```python
from build123d import *

# Parameters (mm, degrees)
BOSS_EXTRUDE1_DEPTH      = 85
BOSS_EXTRUDE1_DEPTH_BACK = 30
CUT_EXTRUDE1_DEPTH       = 134.120246394
CUT_EXTRUDE1_DEPTH_BACK  = 134.120246394
SKETCH3_R                = 20
CHAMFER1_SIZE            = 10
CHAMFER2_SIZE            = 60


with BuildPart() as part:
    # Sketch2 → Boss-Extrude1 (new, two sides: drawn at the far end of the back side and taken through both)
    with BuildSketch(Plane.XY.offset(-BOSS_EXTRUDE1_DEPTH_BACK)):
        Polygon((0, 0), (-50, 0), (-50, 80), (-64, 80), (-64, -8), (14, -8), (14, 80), (0, 80), align=None)
    extrude(amount=BOSS_EXTRUDE1_DEPTH + BOSS_EXTRUDE1_DEPTH_BACK)

    # Sketch3 → Cut-Extrude1 (cut, two sides: drawn at the far end of the back side and taken through both)
    with BuildSketch(Plane(origin=(0, 0, 0), x_dir=(0, 0, -1), z_dir=(1, 0, 0)).offset(-CUT_EXTRUDE1_DEPTH_BACK)):
        with Locations(Location((0, 50, 0), (0, 0, 90))):
            Circle(SKETCH3_R)
    extrude(amount=CUT_EXTRUDE1_DEPTH + CUT_EXTRUDE1_DEPTH_BACK, mode=Mode.SUBTRACT)

    # Chamfer1
    chamfer1_edges = [part.edges().sort_by_distance(p)[0] for p in [
        (-50, 0, 27.5),
        (0, 0, 27.5),
    ]]
    chamfer(chamfer1_edges, length=CHAMFER1_SIZE)

    # Chamfer2
    chamfer2_edges = [part.edges().sort_by_distance(p)[0] for p in [
        (-57, 80, 85),
        (7, 80, 85),
    ]]
    chamfer(chamfer2_edges, length=CHAMFER2_SIZE)


solid = part.part
```
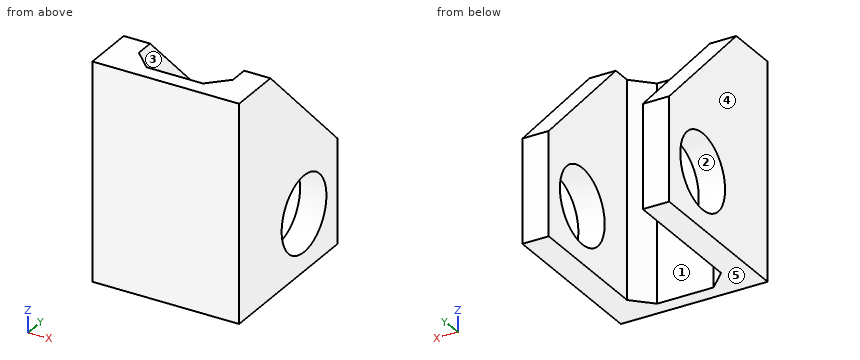
Design review of the part built by this model. Coordinates are the model's own, in mm. Face numbers are marked on the shaded views. A direction names the side the tool comes from. Give positions to 0.01 mm unless a question says otherwise; leave off trailing zeros. Write each loop counter-clockwise with the first axis right and the second up, starting at its lowest first coordinate (ties: lowest second). Pieces come first, ordered by that corner, then holes. Notation, with made-up numbers: (53.5, 31) - (78.5, 31) arc R32 cw to (78.5, 58) - close; hole circle Ø8 at (47.25, 11.5). An arc over 180 degrees is marked (long way). Return JSON: item names as keys, results as strings. Group by question number.
(1) To check wall thickness, follow probe 1 along Y at (x, z) = (-60, 0); probe 2 along X at (y, z) = (17, 46); probe 3 along Y at (x, z) = (-12.5, 53.5). State the ranges of each line that lie inside material, in increasing order.
(2) We need section B-B, the plane y = 50. Give the boundary of the cut face in (x, z).
(3) Mouldability with a two-part tool opening along X and no side actions: class the marked faces 3, 4 and 5 as +X half, -X half, draft (parallel to the pull), parting line (faces both ways), or undercut.
(4) We need section C-C, the plane z = -16. Give the boundary of the cut face in (x, y), then the cut area to 3 significant figures.
(5) Machinability: for the marked faces 1 and 2, which of the approach directions +Z, -Z, +X, -X, +Y, -Y give a long, thin tool a straight path to every point of the face, cutting with its end or side? Answer none if there is none.
(6) Insertion check: pin 1 (12 mm diameter, centred on x = -49, y = 48, fed in from +Z); pin 2 (12 mm diameter, centred on x = -15.5, z = 64.5, fed in from +Y); pin 3 (15 mm diameter, centred on x = -23, z = 9.5, fed in from +Y). Each pin has a flat end and moves straight along its axis. Give the tip position at first contact, or say it passes through.
(7) We need section A-A, the plane z = 0. Give the boundary of the cut face in (x, y).
(8) We need section D-D, the plane x = -52.5. Give the boundary of the cut face in (y, z).
Reported:
{
 "1": {"probe 1": "y = -8 to 30, 70 to 80", "probe 2": "x = -64 to -50, 0 to 14", "probe 3": "y = -8 to 0"},
 "2": {"outline": "(-64, -30) - (-50, -30) - (-50, -20) - (-64, -20) - close; (-64, 20) - (-50, 20) - (-50, 55) - (-64, 55) - close; (0, -30) - (14, -30) - (14, -20) - (0, -20) - close; (0, 20) - (14, 20) - (14, 55) - (0, 55) - close"},
 "3": {"face 3": "undercut", "face 4": "-X half", "face 5": "draft"},
 "4": {"outline": "(-64, -8) - (14, -8) - (14, 38) - (0, 38) - (0, 10) - (-10, 0) - (-40, 0) - (-50, 10) - (-50, 38) - (-64, 38) - close; (-64, 62) - (-50, 62) - (-50, 80) - (-64, 80) - close; (0, 62) - (14, 62) - (14, 80) - (0, 80) - close", "area": "2,290 mm2"},
 "5": {"face 1": "+Z, -Z, +Y", "face 2": "+X, -X"},
 "6": {"pin 1": "stops at z = 62.92", "pin 2": "stops at y = 0.5", "pin 3": "stops at y = 0"},
 "7": {"outline": "(-64, -8) - (14, -8) - (14, 30) - (0, 30) - (0, 10) - (-10, 0) - (-40, 0) - (-50, 10) - (-50, 30) - (-64, 30) - close; (-64, 70) - (-50, 70) - (-50, 80) - (-64, 80) - close; (0, 70) - (14, 70) - (14, 80) - (0, 80) - close"},
 "8": {"outline": "(-8, -30) - (80, -30) - (80, 25) - (20, 85) - (-8, 85) - close; hole circle Ø40 at (50, 0)"}
}
